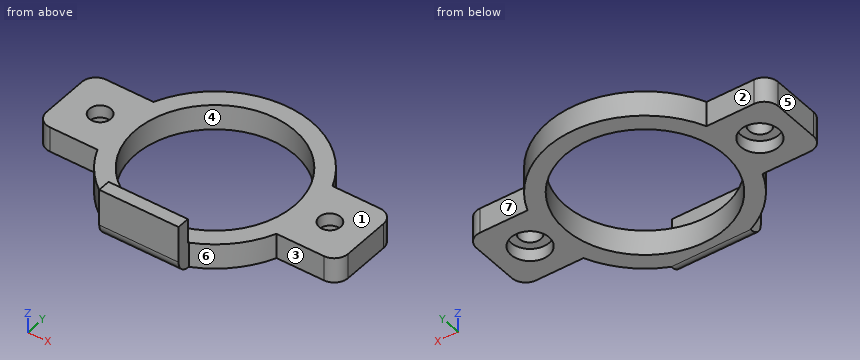
```python
from build123d import *

# Parameters (mm, degrees)
SKETCH_1_R          = 6.344055944
EXTRUDE_2_DEPTH     = 2
SKETCH_1_7_W        = 6.308806274
SKETCH_1_7_H        = 1
EXTRUDE_3_DEPTH     = 4
SKETCH_1_8_R        = 0.855944056
CUT_EXTRUDE_3_DEPTH = 3.5
SKETCH_1_9_R        = 1.51048951
CUT_EXTRUDE_4_DEPTH = 1
FILLET_2_R          = 1.1
FILLET_3_R          = 1.1


with BuildPart() as part:
    # Sketch 1 → Extrude 2 (new body)
    with BuildSketch(Plane.XY):
        with BuildLine():
            Line((3.154403137, -7.15), (-3.154403137, -7.15))
            Line((-3.154403137, -7.15), (-3.154403137, -7.053623266))
            ThreePointArc((-3.154403137, -7.053623266), (-5.522881331, -5.403854378), (-7.120664318, -3))
            Line((-7.120664318, -3), (-12, -3))
            Line((-12, -3), (-12, 3))
            Line((-12, 3), (-7.120664318, 3))
            ThreePointArc((-7.120664318, 3), (0, 7.726827314), (7.120664318, 3))
            Line((7.120664318, 3), (12, 3))
            Line((12, 3), (12, -3))
            Line((12, -3), (7.120664318, -3))
            ThreePointArc((7.120664318, -3), (5.522881331, -5.403854378), (3.154403137, -7.053623266))
            Line((3.154403137, -7.053623266), (3.154403137, -7.15))
        make_face()
        Circle(SKETCH_1_R, mode=Mode.SUBTRACT)
    extrude(amount=EXTRUDE_2_DEPTH)

    # Sketch 1_7 → Extrude 3 (add)
    with BuildSketch(Plane.XY):
        with Locations((0, -7.65)):
            Rectangle(SKETCH_1_7_W, SKETCH_1_7_H)
    extrude(amount=EXTRUDE_3_DEPTH)

    # Sketch 1_8 → Cut-Extrude 3 (cut)
    with BuildSketch(Plane.XY):
        with Locations((-9.139979315, 0)):
            Circle(SKETCH_1_8_R)
        with Locations(Location((9.139979315, 0, 0), (0, 0, 180))):
            Circle(SKETCH_1_8_R)
    extrude(amount=CUT_EXTRUDE_3_DEPTH, mode=Mode.SUBTRACT)

    # Sketch 1_9 → Cut-Extrude 4 (cut)
    with BuildSketch(Plane.XY):
        with Locations((-9.139979315, 0)):
            Circle(SKETCH_1_9_R)
        with Locations(Location((9.139979315, 0, 0), (0, 0, 180))):
            Circle(SKETCH_1_9_R)
    extrude(amount=CUT_EXTRUDE_4_DEPTH, mode=Mode.SUBTRACT)

    # Fillet 2
    fillet_2_edges = [part.edges().sort_by_distance(p)[0] for p in [
        (0, -8.15, 0),
    ]]
    fillet(fillet_2_edges, radius=FILLET_2_R)

    # Fillet 3
    fillet_3_edges = [part.edges().sort_by_distance(p)[0] for p in [
        (12, -3, 1),
        (12, 3, 1),
        (-12, 3, 1),
        (-12, -3, 1),
    ]]
    fillet(fillet_3_edges, radius=FILLET_3_R)


solid = part.part
```
CAD build for the part. Positions are in the model's coordinates, mm. Face numbers are marked on the shaded views. A direction names the side the tool comes from. Coordinates: 2 decimals unless noted, no trailing zeros. Write each loop counter-clockwise with the first axis right and the second up, starting at its lowest first coordinate (ties: lowest second). Pieces come first, ordered by that corner, then holes. Notation, with made-up numbers: (33.5, -10.5) -> (88.5, -10.5) arc R20 cw to (88.5, 4.5) -> close; hole circle Ø11 at (-16.5, 71). An arc over 180 degrees is marked (long way). Return JSON: item names as keys, results as strings. Group by question number.
Q1. Flat gauge pins, fed straight in: pin 1 (1 mm diameter, centred on x = -1, z = 3, fed in from +Y); pin 2 (2 mm diameter, centred on x = -8.5, z = 1, fed in from -Y); pin 3 (1.2 mm diameter, centred on y = -8, z = 2.5, fed in from -X); pin 4 (1.5 mm diameter, centred on x = -9.14, y = 0, fed in from +Z). Where does each tip first touch, or does it go through?
Q2. Cut at C-C, the plane z = 0.6. Give the cut face in (x, y).
Q3. Cut at D-D, the plane y = -0.25. Give the cut face in (x, z).
Q4. Cut at A-A, the plane x = 0. Give the cut face in (y, z), then the cut area to 3 significant figures.
Q5. Which spindle directions (+Z, -Z, +X, -X, +Y, -Y) get a long thin tool onto all of the face, cutting with end or side? Do the marked faces 1, 2 and 3. Say none if no direction does.
Q6. Cut at B-B, the plane y = 2.5. Give the cut face in (x, z).
Q7. Pull direction Y, two halves, no side cores. Call the marked faces 4, 5, 6 and 7: released by +Y, released by -Y, zero draft, split by the parting line, or undercut.
Q8. Drill centre lines: line 1 (Z direction, x = 2.5, y = -6.5); line 2 (Y direction, x = 2.25, z = 3.3); line 3 (X direction, y = 4, z = 1.3). Where is each one in solid material? Low to high.
Returned:
{
 "1": {"pin 1": "stops at y = -7.15", "pin 2": "stops at y = -3", "pin 3": "stops at x = -3.15", "pin 4": "passes through"},
 "2": {"outline": "(-12, -1.9) arc R1.1 ccw to (-10.9, -3) -> (-7.12, -3) arc R7.73 ccw to (-3.15, -7.05) -> (-3.15, -8.03) -> (3.15, -8.03) -> (3.15, -7.05) arc R7.73 ccw to (7.12, -3) -> (10.9, -3) arc R1.1 ccw to (12, -1.9) -> (12, 1.9) arc R1.1 ccw to (10.9, 3) -> (7.12, 3) arc R7.73 ccw to (-7.12, 3) -> (-10.9, 3) arc R1.1 ccw to (-12, 1.9) -> close; hole circle Ø3.02 at (-9.14, 0); hole circle Ø12.69 at (0, 0); hole circle Ø3.02 at (9.14, 0)"},
 "3": {"outline": "(-12, 0) -> (-10.63, 0) -> (-10.63, 1) -> (-9.96, 1) -> (-9.96, 2) -> (-12, 2) -> close; (-8.32, 1) -> (-7.65, 1) -> (-7.65, 0) -> (-6.34, 0) -> (-6.34, 2) -> (-8.32, 2) -> close; (6.34, 0) -> (7.65, 0) -> (7.65, 1) -> (8.32, 1) -> (8.32, 2) -> (6.34, 2) -> close; (9.96, 1) -> (10.63, 1) -> (10.63, 0) -> (12, 0) -> (12, 2) -> (9.96, 2) -> close"},
 "4": {"outline": "(-8.15, 1.1) arc R1.1 ccw to (-7.05, 0) -> (-6.34, 0) -> (-6.34, 2) -> (-7.15, 2) -> (-7.15, 4) -> (-8.15, 4) -> close; (6.34, 0) -> (7.73, 0) -> (7.73, 2) -> (6.34, 2) -> close", "area": "8.12 mm2"},
 "5": {"face 1": "+Z, +X, -X, +Y", "face 2": "+Z, -Z, -X, +Y", "face 3": "+Z, -Z, +X, -Y"},
 "6": {"outline": "(-11.82, 0) -> (-5.83, 0) -> (-5.83, 2) -> (-11.82, 2) -> close; (5.83, 0) -> (11.82, 0) -> (11.82, 2) -> (5.83, 2) -> close"},
 "7": {"face 4": "undercut", "face 5": "zero draft", "face 6": "released by -Y", "face 7": "released by +Y"},
 "8": {"line 1": "z = 0 to 2", "line 2": "y = -8.15 to -7.15", "line 3": "x = -6.61 to -4.92, 4.92 to 6.61"}
}
